Could you check a few things on this model? Use its own coordinates, in mm. Face numbers are marked on the shaded views. A direction names the side the tool comes from. Give positions to 0.01 mm unless a question says otherwise; leave off trailing zeros. Loops run counter-clockwise (first coordinate to the right, second up) from the corner with the lowest first, then second, coordinate; pieces in that order, holes last. Notation, with made-up numbers: (-36, 10) - (23, 10) arc R10 ccw to (23, 29) - close; hole circle Ø11 at (-11.5, 70.5). An arc over 180 degrees is marked (long way). Use CSV: the item, a comma, the result in double quotes.
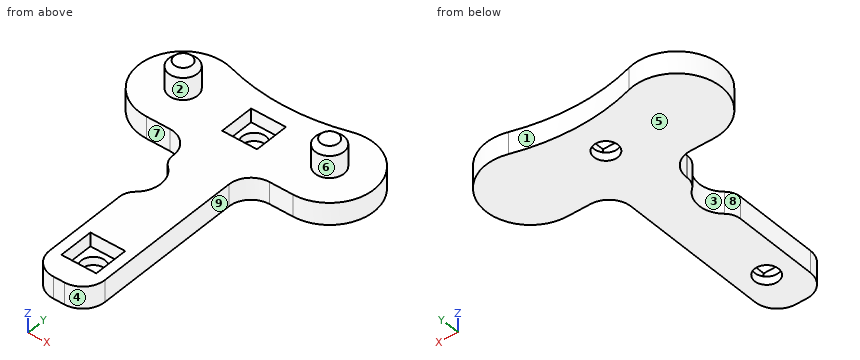
from build123d import *

# Parameters (mm, degrees)
PAD015_DEPTH    = 4
SKETCH023_R     = 2.6
PAD016_DEPTH    = 5
SKETCH024_R     = 2.15
POCKET009_DEPTH = 4.001
SKETCH025_W     = 6.3
SKETCH025_H     = 6.3
POCKET010_DEPTH = 2.5
FILLET007_R     = 4
CHAMFER003_SIZE = 1
SKETCH026_R     = 4.65
POCKET011_DEPTH = 4.001
FILLET008_R     = 3


with BuildPart() as part:
    # Sketch022 → Pad015 (new body)
    with BuildSketch(Plane.XY):
        with BuildLine():
            ThreePointArc((-10.894444, -35.359738), (0, -37), (10.894444, -35.359738))
            ThreePointArc((13.25, -51.005087), (21.16084, -41.814035), (10.894444, -35.359738))
            Line((13.25, -51.005087), (5, -51.005087))
            Line((5, -51.005087), (5, -86.005087))
            Line((-5, -86.005087), (5, -86.005087))
            Line((-5, -51.005087), (-5, -86.005087))
            Line((-13.25, -51.005087), (-5, -51.005087))
            ThreePointArc((-10.894444, -35.359738), (-21.16084, -41.814035), (-13.25, -51.005087))
        make_face()
    extrude(amount=PAD015_DEPTH)

    # Sketch023 (on Face10 of Pad015) → Pad016 (join)
    with BuildSketch(Plane.XY.offset(4)):
        with Locations((-13.25, -43.005087)):
            Circle(SKETCH023_R)
        with Locations((13.25, -43.005087)):
            Circle(SKETCH023_R)
    extrude(amount=PAD016_DEPTH)

    # Sketch024 (on Face5 of Pad016) → Pocket009 (cut, through all)
    with BuildSketch(Plane.XY.offset(4)):
        with Locations((0, -43.505087)):
            Circle(SKETCH024_R)
        with Locations((0, -78.505087)):
            Circle(SKETCH024_R)
    extrude(amount=-POCKET009_DEPTH, mode=Mode.SUBTRACT)

    # Sketch025 (on Face5 of Pocket009) → Pocket010 (cut)
    with BuildSketch(Plane.XY.offset(4)):
        with Locations((0, -43.505087)):
            Rectangle(SKETCH025_W, SKETCH025_H)
        with Locations((0, -78.505087)):
            Rectangle(SKETCH025_W, SKETCH025_H)
    extrude(amount=-POCKET010_DEPTH, mode=Mode.SUBTRACT)

    # Fillet007
    fillet007_edges = [part.edges().sort_by_distance(p)[0] for p in [
        (5, -51.005087, 2),
        (-5, -51.005087, 2),
        (-5, -86.005087, 2),
        (5, -86.005087, 2),
    ]]
    fillet(fillet007_edges, radius=FILLET007_R)

    # Chamfer003
    chamfer003_edges = [part.edges().sort_by_distance(p)[0] for p in [
        (-15.85, -43.005087, 9),
        (10.65, -43.005087, 9),
    ]]
    chamfer(chamfer003_edges, length=CHAMFER003_SIZE)

    # Sketch026 (on Face3 of Chamfer003) → Pocket011 (cut, through all)
    with BuildSketch(Plane.XY.offset(4)):
        with Locations((-7, -61.005087)):
            Circle(SKETCH026_R)
    extrude(amount=-POCKET011_DEPTH, mode=Mode.SUBTRACT)

    # Fillet008
    fillet008_edges = [part.edges().sort_by_distance(p)[0] for p in [
        (-5, -56.807171, 2),
        (-5, -65.203003, 2),
    ]]
    fillet(fillet008_edges, radius=FILLET008_R)


solid = part.part
1) Suppose I cut it at C-C (y = -69.5). Please give me the cut outline in (x, z).
Answer below:
outline,"(-5, 0) - (5, 0) - (5, 4) - (-5, 4) - close"
2) Suppose I cut it at A-A (x = 0). Please give me the cut outline in (y, z), plus the area to 3 significant figures.
Answer below:
outline,"(-86.01, 0) - (-80.66, 0) - (-80.66, 1.5) - (-81.66, 1.5) - (-81.66, 4) - (-86.01, 4) - close; (-76.36, 0) - (-45.66, 0) - (-45.66, 1.5) - (-46.66, 1.5) - (-46.66, 4) - (-75.36, 4) - (-75.36, 1.5) - (-76.36, 1.5) - close; (-41.36, 0) - (-37, 0) - (-37, 4) - (-40.36, 4) - (-40.36, 1.5) - (-41.36, 1.5) - close"
area,"152 mm2"
3) I'm going to push flat-ended pins straight in: P1, Ø3, axis at x = -1.5, y = -77, coming from the +Z side; P2, Ø12, axis at x = -10.5, y = -69, coming from the +Z side; P3, Ø2, axis at y = -65, z = 1.5, coming from the +X side. Where does each tip first touch, or does it pass through?
Answer below:
P1,"stops at z = 1.5"
P2,"stops at z = 4"
P3,"stops at x = 5"
4) Suppose I cut it at D-D (z = 6). Please give me the cut outline in (x, y).
Answer below:
outline,"circle Ø5.2 at (-13.25, -43.01); circle Ø5.2 at (13.25, -43.01)"
5) Suppose I cut it at B-B (z = 2.5). Please give me the cut outline in (x, y), plus the area to 3 significant figures.
Answer below:
outline,"(-13.25, -51.01) - (-9, -51.01) arc R4 cw to (-5, -55.01) - (-5, -55.22) arc R3 ccw to (-3.96, -57.49) arc R4.65 cw to (-3.96, -64.52) arc R3 ccw to (-5, -66.79) - (-5, -82.01) arc R4 ccw to (-1, -86.01) - (1, -86.01) arc R4 ccw to (5, -82.01) - (5, -55.01) arc R4 cw to (9, -51.01) - (13.25, -51.01) arc R8 ccw (long way) to (10.89, -35.36) arc R37 cw to (-10.89, -35.36) arc R8 ccw (long way) to start; hole (-3.15, -81.66) - (3.15, -81.66) - (3.15, -75.36) - (-3.15, -75.36) - close; hole (-3.15, -46.66) - (3.15, -46.66) - (3.15, -40.36) - (-3.15, -40.36) - close"
area,"847 mm2"
6) I need wall thicknesses on line 1 along Y through (x, z) = (0, 1.1); line 2 along Y through (x, z) = (-0.5, 2.75); line 3 along X through (y, z) = (-76.5, 3.75). Which ranges of each line are inside material? Lowest first, please.
Answer below:
line 1,"y = -86.01 to -80.66, -76.36 to -45.66, -41.36 to -37"
line 2,"y = -86.01 to -81.66, -75.36 to -46.66, -40.36 to -37"
line 3,"x = -5 to -3.15, 3.15 to 5"
7) Which directions (+Z, -Z, +X, -X, +Y, -Y) give clear straight access to the entire face, cutting with the end or side of a thin tool? Please do the marked faces 5, 6, 7, 8 and 9.
Answer below:
face 5,"-Z, +X, -X, +Y, -Y"
face 6,"+Z"
face 7,"+Z, -Z, -X, -Y"
face 8,"+Z, -Z, -X"
face 9,"+Z, -Z, +X, -Y"
8) We'd pull the mould along X, two halves only. Please class the marked faces 1, 2, 3 and 4: +X half, -X half, draft (parallel to the pull), parting line (faces both ways), or undercut.
Answer below:
face 1,"undercut"
face 2,"undercut"
face 3,"-X half"
face 4,"+X half"
